The model under review builds one solid part; all positions refer to its coordinate system, in mm. Face numbers are marked on the shaded views. A direction names the side the tool comes from. Round coordinates to 2 decimals unless told otherwise and drop trailing zeros. Loops run counter-clockwise (first coordinate to the right, second up) from the corner with the lowest first, then second, coordinate; pieces in that order, holes last. Notation, with made-up numbers: (9, 39.5) -> (52, 39.5) arc R22 ccw to (52, 57.5) -> close; hole circle Ø6 at (-40, -26). An arc over 180 degrees is marked (long way). Use a Markdown table: item, result. Add a question column.
1) Consider section A-A on x = 3. Give the boundary of the cut face in (y, z).
2) Consider section C-C on z = 3.6. Give the boundary of the cut face in (x, y).
3) Consider section B-B on y = -0.25. Give the boundary of the cut face in (x, z).
4) For the marked faces 4 and 5, list the 3-axis set-ups (+Z, -Z, +X, -X, +Y, -Y) from which the entire face can be reached by the end or side of a thin tool; tool diameter is ignored.
5) Mouldability with a two-part tool opening along Z and no side actions: class the marked faces 1, 2 and 3 as released by +Z, released by -Z, zero draft, split by the parting line, or undercut.
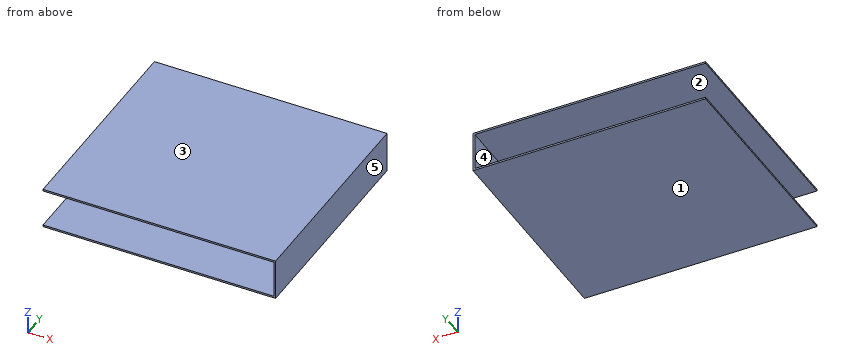
from build123d import *

# Parameters (mm, degrees)
BOX058_W               = 6
BOX058_H               = 6.45
BOX058_DEPTH           = 1.05
BOX057_W               = 6
BOX057_H               = 6.5
BOX057_DEPTH           = 1.15
CUT009_PLACEMENT_ANGLE = 270


with BuildPart() as small_cu_gnd_electrode014:
    # Box058 → Box058 (new body)
    with BuildSketch(Plane.XY.offset(0.05)):
        with Locations((3, 3.225)):
            Rectangle(BOX058_W, BOX058_H)
    extrude(amount=BOX058_DEPTH)


with BuildPart() as small_cu_electrode002_short_axis_gnd:
    # Box057 → Box057 (new body)
    with BuildSketch(Plane.XY):
        with Locations((3, 3.25)):
            Rectangle(BOX057_W, BOX057_H)
    extrude(amount=BOX057_DEPTH)

    # Cut009: cut Small Cu GND Electrode014
    add(small_cu_gnd_electrode014.part, mode=Mode.SUBTRACT)


with BuildPart() as small_cu_electrode002_short_axis_gnd_1:
    # Cut009 placement: moved
    add(small_cu_electrode002_short_axis_gnd.part.moved(Location((-2.38, 3.62, 2.74))).rotate(Axis((-2.38, 3.62, 2.74), (0, 0, 1)), CUT009_PLACEMENT_ANGLE))


solid = small_cu_electrode002_short_axis_gnd_1.part
Result set:
| question | item | result |
|---|---|---|
| 1 | outline | (-2.38, 2.74) -> (3.62, 2.74) -> (3.62, 2.79) -> (-2.38, 2.79) -> close; (-2.38, 3.84) -> (3.62, 3.84) -> (3.62, 3.89) -> (-2.38, 3.89) -> close |
| 2 | outline | (4.07, -2.38) -> (4.12, -2.38) -> (4.12, 3.62) -> (4.07, 3.62) -> close |
| 3 | outline | (-2.38, 2.74) -> (4.12, 2.74) -> (4.12, 3.89) -> (-2.38, 3.89) -> (-2.38, 3.84) -> (4.07, 3.84) -> (4.07, 2.79) -> (-2.38, 2.79) -> close |
| 4 | face 4 | -X, +Y, -Y |
| 4 | face 5 | +Z, -Z, +X, +Y, -Y |
| 5 | face 1 | released by -Z |
| 5 | face 2 | undercut |
| 5 | face 3 | released by +Z |
